Part model, mm, in its own coordinate system. A direction names the side the tool comes from. Give positions to 0.01 mm unless a question says otherwise; leave off trailing zeros. Write each loop counter-clockwise with the first axis right and the second up, starting at its lowest first coordinate (ties: lowest second). Pieces come first, ordered by that corner, then holes. Notation, with made-up numbers: M 30.25,-15.5 L 67.25,-15.5 A33 cw 67.25,12.5 Z; hole C 7.25,33 d8. An arc over 180 degrees is marked long. Use a Markdown table: item, result. Add a question column.
from build123d import *

# Parameters (mm, degrees)
ESQUISSE1_R      = 2.5
EXTRUSION1_DEPTH = 3


with BuildPart() as part:
    # Esquisse1 → Extrusion1 (new body)
    with BuildSketch(Plane.XY):
        with BuildLine():
            Line((150, 292), (-150, 292))
            Line((-150, 292), (-150, 30))
            ThreePointArc((-150, 30), (-135.857864376, 24.142135624), (-130, 10))
            Line((-130, 10), (-130, 0))
            Line((-130, 0), (130, 0))
            Line((130, 0), (130, 10))
            ThreePointArc((130, 10), (135.857864376, 24.142135624), (150, 30))
            Line((150, 30), (150, 292))
        make_face()
        with Locations((134, 277)):
            Circle(ESQUISSE1_R, mode=Mode.SUBTRACT)
        with Locations((-134, 277)):
            Circle(ESQUISSE1_R, mode=Mode.SUBTRACT)
        with Locations((114, 12)):
            Circle(ESQUISSE1_R, mode=Mode.SUBTRACT)
        with Locations((-114, 12)):
            Circle(ESQUISSE1_R, mode=Mode.SUBTRACT)
        with BuildLine():
            Line((-25, 137), (-25, 147))
            ThreePointArc((-25, 147), (0, 172), (25, 147))
            Line((25, 147), (25, 137))
            ThreePointArc((25, 137), (0, 112), (-25, 137))
        make_face(mode=Mode.SUBTRACT)
        with BuildLine():
            Line((-90, 267), (-90, 277))
            ThreePointArc((-90, 277), (-80, 287), (-70, 277))
            Line((-70, 277), (-70, 267))
            ThreePointArc((-70, 267), (-80, 257), (-90, 267))
        make_face(mode=Mode.SUBTRACT)
    extrude(amount=EXTRUSION1_DEPTH)


solid = part.part
1. Cut at B-B (z = 1.15). Write the cut outline in (x, y), then the cut area to 3 significant figures.
2. Cut at C-C (y = 141). Write the cut outline in (x, z), then the cut area to 3 significant figures.
3. Flat gauge pin, fed straight in: pin 1 (4 mm diameter, centred on x = -114, y = 12, fed in from -Z). Where does the tip first touch, or does it go through?
4. Mould opens along Y. For faces 1 (the flat face through (31, 148, 3)), 2 (the cylindrical face through (0.55, 112.006, 1.479)), 3 (the cylindrical face through (-136.014, 24.297, 1.479)) say: released by +Y, released by -Y, zero draft, split by the parting line, or undercut.
5. Drill centre lines: probe 1 along X at (y, z) = (277, 0.85); probe 2 along Y at (x, z) = (114, 1.05); probe 3 along Y at (x, z) = (0, 2.25). Where is each one in solid material? Low to high. Write a range as [from, to].
6. Cut at A-A (x = -80). Write the cut outline in (y, z), then the cut area to 3 significant figures.
7. Tool access for faces 4 (the cylindrical face through (135.703, 23.986, 1.479)), 5 (the cylindrical face through (-80, 257, 1)): list every direction of +Z, -Z, +X, -X, +Y, -Y with a clear straight run to the whole face (end or side of a thin tool).
A:
| question | item | result |
|---|---|---|
| 1 | outline | M -150,30 A20 cw -130,10 L -130,0 L 130,0 L 130,10 A20 cw 150,30 L 150,292 L -150,292 Z; hole C -134,277 d5; hole C -114,12 d5; hole M -90,267 A10 ccw -70,267 L -70,277 A10 ccw -90,277 Z; hole M -25,137 A25 ccw 25,137 L 25,147 A25 ccw -25,147 Z; hole C 114,12 d5; hole C 134,277 d5 |
| 1 | area | 83,500 mm² |
| 2 | outline | M -150,0 L -25,0 L -25,3 L -150,3 Z; M 25,0 L 150,0 L 150,3 L 25,3 Z |
| 2 | area | 750 mm² |
| 3 | pin 1 | passes through |
| 4 | face 1 | zero draft |
| 4 | face 2 | undercut |
| 4 | face 3 | released by -Y |
| 5 | probe 1 | x = [-150, -136.5], [-131.5, -90], [-70, 131.5], [136.5, 150] |
| 5 | probe 2 | y = [0, 9.5], [14.5, 292] |
| 5 | probe 3 | y = [0, 112], [172, 292] |
| 6 | outline | M 0,0 L 257,0 L 257,3 L 0,3 Z; M 287,0 L 292,0 L 292,3 L 287,3 Z |
| 6 | area | 786 mm² |
| 7 | face 4 | +Z, -Z, +X, -Y |
| 7 | face 5 | +Z, -Z |
